from build123d import *

# Parameters (mm, degrees)
F1_DEPTH  = 15
F2_R      = 2.1
F3_DEPTH  = 50.001
F4_W      = 3.5
F4_H      = 7.3
F5_DEPTH  = 13.101
F6_R      = 4.1
F7_DEPTH  = 18.001
F9_DEPTH  = 2
F10_R     = 7.5
F10_R_2   = 6.6
F11_DEPTH = 2


with BuildPart() as f1:
    # F0 (on Top) → F1 (new body)
    with BuildSketch(Plane.XY):
        with BuildLine():
            Line((0, 4.1), (0, 0))
            Line((0, 0), (0, -4.1))
            Line((0, -4.1), (20, -4.1))
            Line((20, -4.1), (20, -8))
            ThreePointArc((20, -8), (20.292893, -8.707107), (21, -9))
            Line((21, -9), (50, -9))
            Line((50, -9), (50, -6))
            Line((50, -6), (23, -6))
            Line((23, -6), (23, 0))
            Line((23, 0), (23, 6))
            Line((23, 6), (50, 6))
            Line((50, 6), (50, 9))
            Line((50, 9), (21, 9))
            ThreePointArc((21, 9), (20.292893, 8.707107), (20, 8))
            Line((20, 8), (20, 4.1))
            Line((20, 4.1), (0, 4.1))
        make_face()
    extrude(amount=F1_DEPTH)

    # F2 (on face) → F3 (cut, through all)
    with BuildSketch(Plane(origin=(0, 0, 0), x_dir=(0, -1, 0), z_dir=(-1, 0, 0))):
        with Locations((0, 7.5)):
            Circle(F2_R)
    extrude(amount=-F3_DEPTH, mode=Mode.SUBTRACT)

    # F4 (on face) → F5 (cut, through all)
    with BuildSketch(Plane.XZ.offset(4.1)):
        with Locations((6.75, 7.5)):
            Rectangle(F4_W, F4_H)
    extrude(amount=-F5_DEPTH, mode=Mode.SUBTRACT)

    # F6 (on face) → F7 (cut, through all)
    with BuildSketch(Plane(origin=(0, 9, 0), x_dir=(-1, 0, 0), z_dir=(0, 1, 0))):
        with Locations((-40, 7.5)):
            Circle(F6_R)
        Polygon((-45.5, 15), (-50, 15), (-50, 10.5), align=None)
        Polygon((-50, 4.5), (-50, 0), (-45.5, 0), align=None)
    extrude(amount=-F7_DEPTH, mode=Mode.SUBTRACT)

    # F8 (on face) → F9 (join)
    with BuildSketch(Plane.XZ.offset(9)):
        Polygon((44.330127, 15), (35.669873, 15), (31.339746, 7.5), (35.669873, 0), (44.330127, 0), (48.660254, 7.5), align=None)
        Polygon((32.378976, 7.5), (36.189488, 14.1), (43.810512, 14.1), (47.621024, 7.5), (43.810512, 0.9), (36.189488, 0.9), align=None, mode=Mode.SUBTRACT)
    extrude(amount=F9_DEPTH)

    # F10 (on face) → F11 (join)
    with BuildSketch(Plane(origin=(0, 9, 0), x_dir=(-1, 0, 0), z_dir=(0, 1, 0))):
        with Locations((-40, 7.5)):
            Circle(F10_R)
        with Locations((-40, 7.5)):
            Circle(F10_R_2, mode=Mode.SUBTRACT)
    extrude(amount=F11_DEPTH)


solid = f1.part
Here's how the part is built. I have some questions about the finished solid (model axes, mm). A direction names the side the tool comes from. Coordinates: 2 decimals unless noted, no trailing zeros. Loops run counter-clockwise (first coordinate to the right, second up) from the corner with the lowest first, then second, coordinate; pieces in that order, holes last.
1. For faces 4 (the flat face through (5, 0, 5)), 5 (the flat face through (33.535, -9.986, 11.302)), 6 (the flat face through (49, -9, 7)), 7 (the flat face through (46.465, -9.986, 3.698)), which set-ups out of +Z, -Z, +X, -X, +Y, -Y let a thin tool reach every point of the face, with its end or its side?
2. For P1, Ø6, axis at y = 1, z = 9, coming from the +X side; P2, Ø6, axis at x = 18, y = -5.5, coming from the -Z side; P3, Ø6.5, axis at x = 39, z = 10, coming from the +Y side; P4, Ø7.5, axis at x = 40, z = 7.5, coming from the +Y side, each with a flat end and sliding along its axis, tell me the tip position at first contact or that it passes through.
3. If we mould it in two halves opening along Z, with no side actions, what happens to faces 1 (the cylindrical face through (36.452, 9.986, 13.065)), 2 (the cylindrical face through (32.846, 9.986, 9.753)), 3 (the cylindrical face through (20.301, 8.715, 7.395))? For each: pulls with the +Z half, pulls with the -Z half, needs draft (parallel to the pull), parting line crosses it, or undercut.
4. Imagine slicing it at B-B, the plane y = -9.5. Please give me the cut outline in (x, z).
5. I need wall thicknesses on L1, parallel to Y at x = 33, z = 14.25; L2, parallel to X at y = 1.75, z = 10.5; L3, parallel to X at y = -5.5, z = 5.5. Which ranges of each line are inside material? Lowest first, please.
6. Imagine slicing it at C-C, the plane x = 24.5. Please give me the cut outline in (y, z), and give its area (3 significant figures).
7. Imagine slicing it at A-A, the plane y = 0. Please give me the cut outline in (x, z), and give its area (3 significant figures).
8. Imagine slicing it at D-D, the plane x = 12. Please give me the cut outline in (y, z), and give its area (3 significant figures).
Taken from the geometry:
1. face 4: +Y, -Y
1. face 5: +Z, -X, -Y
1. face 6: +X, -Y
1. face 7: -Z, +X, -Y
2. P1: stops at x = 23
2. P2: stops at z = 0
2. P3: stops at y = 9
2. P4: passes through
3. face 1: undercut
3. face 2: parting line crosses it
3. face 3: needs draft
4. outline: (31.34, 7.5) - (35.67, 0) - (44.33, 0) - (48.66, 7.5) - (44.33, 15) - (35.67, 15) - close; hole (32.38, 7.5) - (36.19, 0.9) - (43.81, 0.9) - (47.62, 7.5) - (43.81, 14.1) - (36.19, 14.1) - close
5. L1: y = -9 to -6, 6 to 9
5. L2: x = 0 to 5, 8.5 to 23
5. L3: x = 20 to 23
6. outline: (-9, 0) - (-6, 0) - (-6, 15) - (-9, 15) - close; (6, 0) - (9, 0) - (9, 15) - (6, 15) - close
6. area: 90.0 mm2
7. outline: (0, 0) - (23, 0) - (23, 5.4) - (8.5, 5.4) - (8.5, 3.85) - (5, 3.85) - (5, 5.4) - (0, 5.4) - close; (0, 9.6) - (5, 9.6) - (5, 11.15) - (8.5, 11.15) - (8.5, 9.6) - (23, 9.6) - (23, 15) - (0, 15) - close
7. area: 238 mm2
8. outline: (-4.1, 0) - (4.1, 0) - (4.1, 15) - (-4.1, 15) - close; hole circle Ø4.2 at (0, 7.5)
8. area: 109 mm2
